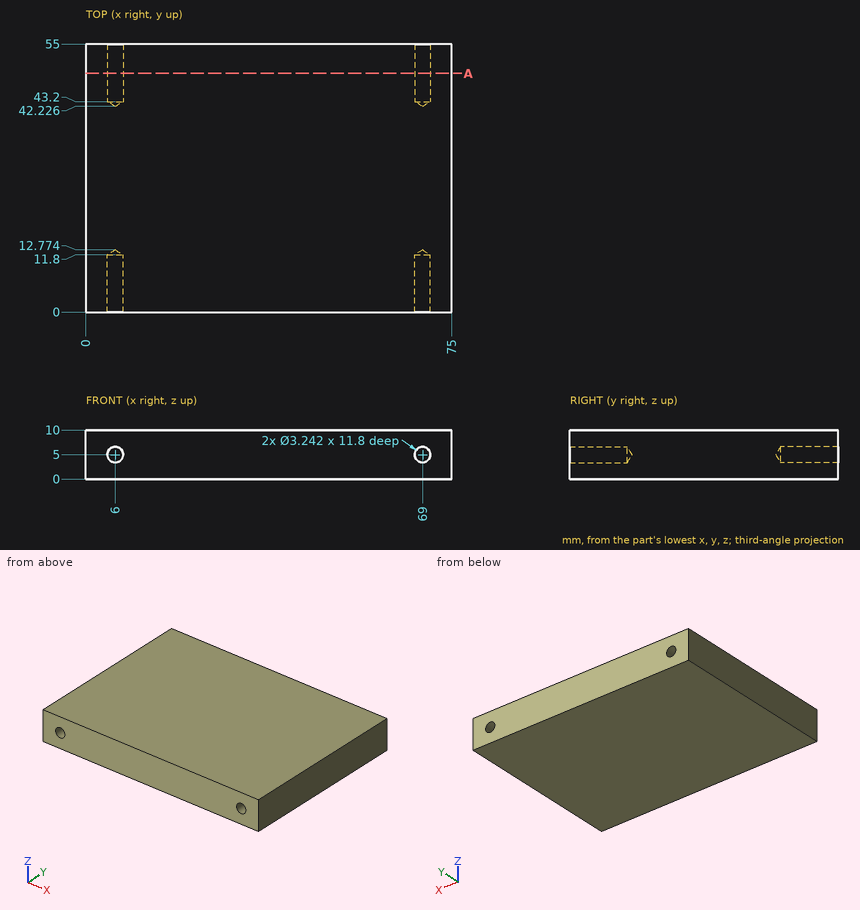
Answer from the drawing. Dimensions are ordinates in mm from the lowest x, y and z of the part. Coordinates: 2 decimals unless noted, no trailing zeros. Loops run counter-clockwise (first coordinate to the right, second up) from the corner with the lowest first, then second, coordinate; pieces in that order, holes last. Notation, with made-up numbers: (19.5, -3.5) - (49.5, -3.5) arc R15 cw to (49.5, 13.5) - close; hole circle Ø9 at (70, -36). An arc over 180 degrees is marked (long way). Answer in a Markdown table with one row per item.
1. Straight lines are drawn through the part: line 1 (X direction, y = 49, z = 5); line 2 (Z direction, x = 6, y = 52); line 3 (X direction, y = 49.5, z = 4.25). For each, find the intervals that lie inside material, in ascending order.
Conclusion:
| item | result |
|---|---|
| line 1 | x = 0 to 4.38, 7.62 to 67.38, 70.62 to 75 |
| line 2 | z = 0 to 3.38, 6.62 to 10 |
| line 3 | x = 0 to 4.56, 7.44 to 67.56, 70.44 to 75 |
2. Find section A-A, the plane y = 49. Write down the section's boundary in (x, z).
Conclusion:
| item | result |
|---|---|
| outline | (0, 0) - (75, 0) - (75, 10) - (0, 10) - close; hole circle Ø3.24 at (6, 5); hole circle Ø3.24 at (69, 5) |
3. Given pin 1 (3 mm diameter, centred on x = 6, z = 5, fed in from -Y); pin 2 (1.9 mm diameter, centred on x = 69, z = 5, fed in from -Y), each flat-ended and moving along its own axis, determine where each tip first touches the part or whether it passes through.
Conclusion:
| item | result |
|---|---|
| pin 1 | stops at y = 11.87 |
| pin 2 | stops at y = 12.2 |
